from build123d import *

# Parameters (mm, degrees)
F0_R        = 9.25
F1_DEPTH    = 5
F3_DEPTH    = 1.2
F4_T1_DEPTH = 12.1393431135
F5_R        = 2


# Not quite as in the source:
# - a fillet or chamfer that OpenCascade refuses, or shapes differently, is made with other operations: its cross-section is extruded or revolved along the edge and cut away or added


with BuildPart() as f1:
    # F0 (on Top) → F1 (new body)
    with BuildSketch(Plane.XY):
        Circle(F0_R)
    extrude(amount=F1_DEPTH)

    # F2 (on face) → F3 (join)
    with BuildSketch(Plane(origin=(0, 0, 0), x_dir=(1, 0, 0), z_dir=(0, 0, -1))):
        with BuildLine():
            Line((-6, 7.0400639202), (-6, 8.8594582227))
            ThreePointArc((-6, 8.8594582227), (-10.7, 0), (-6, -8.8594582227))
            Line((-6, -8.8594582227), (-6, -7.0400639202))
            ThreePointArc((-6, -7.0400639202), (-9.25, 0), (-6, 7.0400639202))
        make_face()
        with BuildLine():
            Line((-6, -7.0400639202), (-6, 7.0400639202))
            ThreePointArc((-6, 7.0400639202), (-9.25, 0), (-6, -7.0400639202))
        make_face()
        with BuildLine():
            Line((6, -7.0400639202), (6, 7.0400639202))
            ThreePointArc((6, 7.0400639202), (0, 9.25), (-6, 7.0400639202))
            Line((-6, 7.0400639202), (-6, -7.0400639202))
            ThreePointArc((-6, -7.0400639202), (0, -9.25), (6, -7.0400639202))
        make_face()
        with BuildLine():
            ThreePointArc((9.25, 0), (8.3982885161, 3.8770156048), (6, 7.0400639202))
            Line((6, 7.0400639202), (6, -7.0400639202))
            ThreePointArc((6, -7.0400639202), (8.3982885161, -3.8770156048), (9.25, 0))
        make_face()
        with BuildLine():
            ThreePointArc((6, -8.8594582227), (9.4522484098, -5.0144790358), (10.7, 0))
            ThreePointArc((10.7, 0), (9.4522484098, 5.0144790358), (6, 8.8594582227))
            Line((6, 8.8594582227), (6, 7.0400639202))
            ThreePointArc((6, 7.0400639202), (8.3982885161, 3.8770156048), (9.25, 0))
            ThreePointArc((9.25, 0), (8.3982885161, -3.8770156048), (6, -7.0400639202))
            Line((6, -7.0400639202), (6, -8.8594582227))
        make_face()
    extrude(amount=-F3_DEPTH)

    # F4: fillet of radius 1 on 4 edges, made by hand

    # F4_s2 → F4_t1 (cut)
    with BuildSketch(Plane.XY.offset(-5.4696715568)):
        with BuildLine():
            ThreePointArc((6, -7.0400639202), (6.7195608847, -7.728089766), (7.6766055002, -7.4538398154))
            ThreePointArc((7.6766055002, -7.4538398154), (6.8743236234, -8.1996143032), (6, -8.8594582227))
            Line((6, -8.8594582227), (6, -7.0400639202))
        make_face()
        with BuildLine():
            ThreePointArc((-7.6766055002, -7.4538398154), (-6.7195608847, -7.728089766), (-6, -7.0400639202))
            Line((-6, -7.0400639202), (-6, -8.8594582227))
            ThreePointArc((-6, -8.8594582227), (-6.8743236234, -8.1996143032), (-7.6766055002, -7.4538398154))
        make_face()
        with BuildLine():
            ThreePointArc((7.6766055002, 7.4538398154), (6.7195608847, 7.728089766), (6, 7.0400639202))
            Line((6, 7.0400639202), (6, 8.8594582227))
            ThreePointArc((6, 8.8594582227), (6.8743236234, 8.1996143032), (7.6766055002, 7.4538398154))
        make_face()
        with BuildLine():
            ThreePointArc((-6, 7.0400639202), (-6.7195608847, 7.728089766), (-7.6766055002, 7.4538398154))
            ThreePointArc((-7.6766055002, 7.4538398154), (-6.8743236234, 8.1996143032), (-6, 8.8594582227))
            Line((-6, 8.8594582227), (-6, 7.0400639202))
        make_face()
    extrude(amount=F4_T1_DEPTH, mode=Mode.SUBTRACT)

    # F5
    f5_edges = [f1.edges().sort_by_distance(p)[0] for p in [
        (-9.25, 0, 5),
    ]]
    fillet(f5_edges, radius=F5_R)


solid = f1.part
The model under review builds one solid part; all positions refer to its coordinate system, in mm. A direction names the side the tool comes from. Give positions to 0.01 mm unless a question says otherwise; leave off trailing zeros. Loops run counter-clockwise (first coordinate to the right, second up) from the corner with the lowest first, then second, coordinate; pieces in that order, holes last. Notation, with made-up numbers: (-21.5, 2) -> (16.5, 2) arc R23 cw to (16.5, 16) -> close; hole circle Ø11 at (-21.75, 80.25). An arc over 180 degrees is marked (long way). Write each question's results on one line, items separated by ' | '.
1) For line 1 along Z through (x, y) = (9.75, 4); line 2 along Z through (x, y) = (-5.25, 6.25); line 3 along X through (y, z) = (-7, 3.6), list the stretches that pass through material, from the lowest coordinate up. Write a range as from..to.
Conclusion:
line 1: z = 0..1.2 | line 2: z = 0..4.78 | line 3: x = -5.9..5.9
2) Insertion check: pin 1 Ø2 at (y, z) = (-1, 3) entering from +X; pin 2 Ø1 at (x, z) = (-1, 4) entering from +Y; pin 3 Ø1.5 at (y, z) = (-2, 2.5) entering from -X. Each pin has a flat end and moves straight along its axis. Give the tip position at first contact, or say it passes through.
Conclusion:
pin 1: stops at x = 9.25 | pin 2: stops at y = 9.14 | pin 3: stops at x = -9.17
3) Tool access review of faces 4 (the face through (9.4, 0, 1.2)), 5 (the face through (8.545, -3.543, 1.812)), 6 (the face through (0, 0, 0)), 7 (the face through (-9.4, -0.6, 1.2)): name each direction out of +Z, -Z, +X, -X, +Y, -Y from which nothing blocks a thin tool from reaching the whole face with its end or side.
Conclusion:
face 4: +Z, +X | face 5: +Z | face 6: -Z, +X, -X, +Y, -Y | face 7: +Z, -X
4) Draft analysis for pull direction X (two halves, no side actions). For faces 1 (the face through (6.705, -7.724, 0.592)), 2 (the face through (-10.7, -0.1, 0.6)), 3 (the face through (0, 0, 5)), state which applies: pulls with the +X half, pulls with the -X half, needs draft (parallel to the pull), parting line crosses it, or undercut.
Conclusion:
face 1: undercut | face 2: pulls with the -X half | face 3: needs draft
5) Take a section at C-C, the plane z = 1.85. Give the boundary of the cut face in (x, y), plus the area to 3 significant figures.
Conclusion:
outline: circle Ø18.5 at (0, 0) | area: 269 mm^2
6) Take a section at D-D, the plane z = 4.45. Give the boundary of the cut face in (x, y) (1 decimal).
Conclusion:
outline: circle Ø17.3 at (0, 0)
7) Take a section at A-A, the plane x = 0. Give the boundary of the cut face in (y, z).
Conclusion:
outline: (-9.25, 0) -> (9.25, 0) -> (9.25, 3) arc R2 ccw to (7.25, 5) -> (-7.25, 5) arc R2 ccw to (-9.25, 3) -> close
8) Take a section at B-B, the plane z = 0.75. Give the boundary of the cut face in (x, y).
Conclusion:
outline: (-7.68, -7.45) arc R1 ccw to (-6, -7.04) arc R9.25 ccw to (6, -7.04) arc R1 ccw to (7.68, -7.45) arc R10.7 ccw to (7.68, 7.45) arc R1 ccw to (6, 7.04) arc R9.25 ccw to (-6, 7.04) arc R1 ccw to (-7.68, 7.45) arc R10.7 ccw to start
